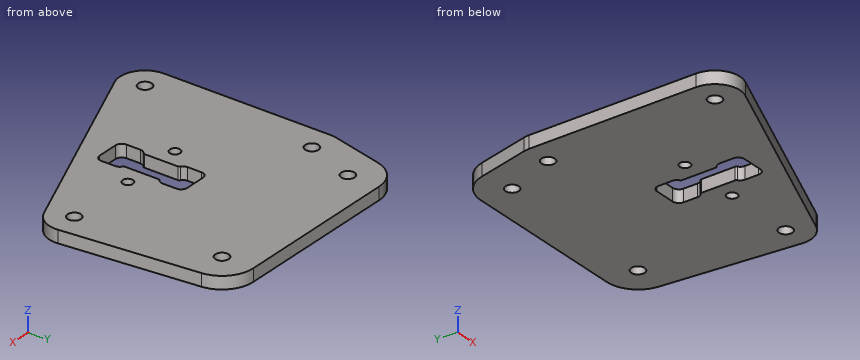
Autodesk Inventor part; units mm, degrees
ref_plane "YZ Plane" through (0, 0, 0) normal (1, 0, 0) x (0, 1, 0)
ref_plane "XZ Plane" through (0, 0, 0) normal (0, 1, 0) x (-1, 0, 0)
ref_plane "XY Plane" through (0, 0, 0) normal (0, 0, 1) x (1, 0, 0)
sketch "スケッチ1" plane through (0, 0, 0) normal (0, 0, 1) x (1, 0, 0)
  line L0 (-15, 61.4764) -> (15, 61.4764) construction
  line L1 (15, 61.4764) -> (15, -42.9448) construction
  line L2 (15, -42.9448) -> (-15, -42.9448) construction
  line L3 (-15, -42.9448) -> (-15, 61.4764) construction
  circle A0 centre (-24.5, 20) radius 9.5 construction
  circle A1 centre (24.5, 0) radius 9.5 construction
  circle A2 centre (-24.5, -20) radius 9.5 construction
  line L4 (-3, 9.5) -> (3, 9.5) construction
  line L5 (3, 9.5) -> (3, -9.5) construction
  line L6 (3, -9.5) -> (-3, -9.5) construction
  line L7 (-3, -9.5) -> (-3, 9.5) construction
  circle A3 centre (-7.5, 0) radius 1.25
  circle A4 centre (7.5, 0) radius 1.25
  circle A5 centre (-20, 32) radius 1.6
  circle A6 centre (20, 32) radius 1.6
  line L8 (-24.5, 20) -> (-24.5, -20) construction
  line L9 (-24.5, -20) -> (24.5, 0) construction
  line L10 (24.5, 0) -> (-24.5, 20) construction
  line L11 (-61.4764, 39.5) -> (49.785, 39.5) construction
  line L12 (49.785, 39.5) -> (49.785, 24.5) construction
  line L13 (49.785, 24.5) -> (-61.4764, 24.5) construction
  line L14 (-61.4764, 24.5) -> (-61.4764, 39.5) construction
  circle A7 centre (-24.5, 20) radius 1.6
  circle A8 centre (24.5, 0) radius 1.6
  circle A9 centre (-24.5, -20) radius 1.6
  arc A10 (-20, 39.5) -> (-27.2824, 33.7934) centre (-20, 32) ccw
  arc A11 (27.4674, 32.6985) -> (20, 39.5) centre (20, 32) ccw
  arc A12 (-30.3259, 21.4347) -> (-30.5, 20) centre (-24.5, 20) ccw
  arc A13 (-30.5, -20) -> (-22.2326, -25.5551) centre (-24.5, -20) ccw
  arc A14 (26.7674, -5.5551) -> (30.4739, 0.5588) centre (24.5, 0) ccw
  line L15 (-20, 39.5) -> (20, 39.5)
  line L16 (-27.2824, 33.7934) -> (-30.3259, 21.4347)
  line L17 (-30.5, 20) -> (-30.5, -20)
  line L18 (-22.2326, -25.5551) -> (26.7674, -5.5551)
  line L19 (30.4739, 0.5588) -> (27.4674, 32.6985)
  line L20 (-2.5, -10.5) -> (2.5, -10.5)
  line L21 (4, -9) -> (4, -5.6703)
  line L22 (2.5, 10.5) -> (-2.5, 10.5)
  line L23 (-3.1, 4) -> (-3.1, -4)
  line L24 (3.1, 4) -> (3.1, -4)
  line L25 (-4, -5.6703) -> (-4, -9)
  line L26 (4, 5.6703) -> (4, 9)
  arc A15 (-2.5, 10.5) -> (-4, 9) centre (-2.5, 9) ccw
  arc A16 (4, 9) -> (2.5, 10.5) centre (2.5, 9) ccw
  arc A17 (-4, -9) -> (-2.5, -10.5) centre (-2.5, -9) ccw
  arc A18 (2.5, -10.5) -> (4, -9) centre (2.5, -9) ccw
  line L27 (-4, 9) -> (-4, 5.6703)
  arc A19 (-4, 5.6703) -> (-3.325, 4.4176) centre (-2.5, 5.6703) ccw
  arc A20 (-3.1, 4) -> (-3.325, 4.4176) centre (-3.6, 4) ccw
  arc A21 (3.325, 4.4176) -> (4, 5.6703) centre (2.5, 5.6703) ccw
  arc A22 (3.325, 4.4176) -> (3.1, 4) centre (3.6, 4) ccw
  arc A23 (-3.325, -4.4176) -> (-4, -5.6703) centre (-2.5, -5.6703) ccw
  arc A24 (-3.325, -4.4176) -> (-3.1, -4) centre (-3.6, -4) ccw
  arc A25 (3.1, -4) -> (3.325, -4.4176) centre (3.6, -4) ccw
  arc A26 (4, -5.6703) -> (3.325, -4.4176) centre (2.5, -5.6703) ccw
  circle A27 centre (-24.5, 20) radius 4 construction
  point P0 (0, 0)
  dimension "d0" = 30
  dimension "d1" = 15
  dimension "d2" = 19
  dimension "d3" = 19
  dimension "d4" = 19
  dimension "d5" = 6
  dimension "d6" = 19
  dimension "d7" = 3
  dimension "d8" = 9.5
  dimension "d9" = 2.5
  dimension "d10" = 2.5
  dimension "d11" = 15
  dimension "d12" = 7.5
  dimension "d13" = 3.2
  dimension "d14" = 3.2
  dimension "d15" = 40
  dimension "d16" = 40
  dimension "d17" = 20
  dimension "d18" = 12
  dimension "d19" = 15
  dimension "d20" = 7.5
  dimension "d21" = 3.2
  dimension "d22" = 3.2
  dimension "d23" = 3.2
  dimension "d24" = 7.5
  dimension "d25" = 7.5
  dimension "d26" = 6
  dimension "d27" = 6
  dimension "d28" = 6
  dimension "d29" = 1
  dimension "d32" = 8
  dimension "d33" = 4
  dimension "d34" = 0.1
  dimension "d35" = 0.1
  dimension "d36" = 1
  dimension "d37" = 1
  dimension "d38" = 1
  dimension "d39" = 1.5
  dimension "d40" = 1
  dimension "d41" = 1.5
  dimension "d42" = 0.5
  dimension "d44" = 1
  dimension "d45" = 1.5
  dimension "d46" = 0.5
  dimension "d47" = 1.5
  dimension "d48" = 0.5
  dimension "d49" = 0.5
  dimension "d50" = 1.5
  dimension "d54" = 8
extrude "押し出し1" add sketch "スケッチ1" along normal blind 3
properties part number "上昇機構_内側板" material "アルミニウム 6061"
Source: CAD feature listing. Evaluate the final solid. Frame: model axes, mm. Round coordinates to 2 decimals unless told otherwise and drop trailing zeros. Loops run counter-clockwise (first coordinate to the right, second up) from the corner with the lowest first, then second, coordinate; pieces in that order, holes last. Notation, with made-up numbers: M 52.5,-38.75 L 93.5,-38.75 A15 cw 93.5,-14.75 Z; hole C 27.5,20 d11. An arc over 180 degrees is marked long. Answer as CSV lines item,"result".
Q1. Cut plane C-C (z = 2.15). Count the separate pieces of the cut face and the enclosed holes in it, plus the area to 3 significant figures.
Verdict:
separate pieces,"1"
enclosed holes,"8"
area,"3,060 mm^2"
Q2. Line query: line 1 along X through (y, z) = (-19.5, 2.35); line 2 along Y through (x, z) = (-20, 1.2); line 3 along X through (y, z) = (10, 1.45). Output: solid intervals per line, ascending.
Verdict:
line 1,"x = -30.5 to -26.02, -22.98 to -7.4"
line 2,"y = -24.64 to 30.4, 33.6 to 39.5"
line 3,"x = -30.5 to -3.62, 3.62 to 29.59"
Q3. Cut plane D-D (y = -13.5). Return the cut outline in (x, z).
Verdict:
outline,"M -30.5,0 L 7.3,0 L 7.3,3 L -30.5,3 Z"
Q4. Contact query for flat-ended pins moving along their axis: pin 1 (1.5 mm diameter, centred on y = -7.5, z = 1, fed in from +X); pin 2 (0.9 mm diameter, centred on y = 7.5, z = 2, fed in from +X). Output: stop coordinate, or through.
Verdict:
pin 1,"stops at x = 23.84"
pin 2,"stops at x = 29.87"
Q5. Cut plane B-B (x = -1). Return the cut outline in (y, z).
Verdict:
outline,"M -16.89,0 L -10.5,0 L -10.5,3 L -16.89,3 Z; M 10.5,0 L 39.5,0 L 39.5,3 L 10.5,3 Z"
Q6. Cut plane A-A (x = -24.5). Return the cut outline in (y, z), plus the area to 3 significant figures.
Verdict:
outline,"M -26,0 L -21.6,0 L -21.6,3 L -26,3 Z; M -18.4,0 L 18.4,0 L 18.4,3 L -18.4,3 Z; M 21.6,0 L 38,0 L 38,3 L 21.6,3 Z"
area,"173 mm^2"
